Work out the finished part from the listing and answer in its coordinate system (mm). Face numbers are marked on the shaded views. A direction names the side the tool comes from. Coordinates: 2 decimals unless noted, no trailing zeros. Loops run counter-clockwise (first coordinate to the right, second up) from the corner with the lowest first, then second, coordinate; pieces in that order, holes last. Notation, with made-up numbers: (69, 2.25) -> (75, 2.25) arc R14 cw to (75, 14.25) -> close; hole circle Ø9 at (-1.5, 44.5). An arc over 180 degrees is marked (long way). One line per question, with ' | ' between items.
```python
from build123d import *

# Parameters (mm, degrees)
BOSS_EXTRUDE3_DEPTH = 25
BOSS_EXTRUDE4_DEPTH = 14
SKETCH9_R           = 14
CUT_EXTRUDE5_DEPTH  = 97
SKETCH10_W          = 12
SKETCH10_H          = 12
CUT_EXTRUDE6_DEPTH  = 97
SKETCH11_R          = 8
BOSS_EXTRUDE5_DEPTH = 14
FILLET3_R           = 14
SKETCH12_R          = 6
CUT_EXTRUDE8_DEPTH  = 54
FILLET4_R           = 3


with BuildPart() as part:
    # Sketch2 → Boss-Extrude3 (new body, symmetric)
    with BuildSketch(Plane.XY):
        with BuildLine():
            Line((0, 0), (55, 0))
            ThreePointArc((55, 0), (78, 23), (101, 0))
            Line((101, 0), (114, 0))
            ThreePointArc((114, 0), (109.720584442, 17.023645986), (97.899748742, 30))
            Line((97.899748742, 30), (58.100251258, 30))
            ThreePointArc((58.100251258, 30), (49.293476177, 21.724076274), (43.721726998, 11))
            Line((43.721726998, 11), (0, 11))
            Line((0, 11), (0, 0))
        make_face()
    extrude(amount=BOSS_EXTRUDE3_DEPTH, both=True)

    # Sketch7 → Boss-Extrude4 (add, symmetric)
    with BuildSketch(Plane.XY):
        with BuildLine():
            Line((114, 0), (114, 72))
            ThreePointArc((114, 72), (95, 91), (76, 72))
            Line((76, 72), (76, 35.944401511))
            ThreePointArc((76, 35.944401511), (66.65391142, 34.165278777), (58.100251258, 30))
            Line((58.100251258, 30), (97.899748742, 30))
            ThreePointArc((97.899748742, 30), (109.720584442, 17.023645986), (114, 0))
        make_face()
    extrude(amount=BOSS_EXTRUDE4_DEPTH, both=True)

    # Sketch9 → Cut-Extrude5 (cut)
    with BuildSketch(Plane.XY.offset(14)):
        with Locations((95, 72)):
            Circle(SKETCH9_R)
    extrude(amount=-CUT_EXTRUDE5_DEPTH, mode=Mode.SUBTRACT)

    # Sketch10 → Cut-Extrude6 (cut)
    with BuildSketch(Plane(origin=(114, 0, 0), x_dir=(0, 0, -1), z_dir=(1, 0, 0))):
        with Locations((0, 85)):
            Rectangle(SKETCH10_W, SKETCH10_H)
    extrude(amount=-CUT_EXTRUDE6_DEPTH, mode=Mode.SUBTRACT)

    # Sketch11 → Boss-Extrude5 (add)
    with BuildSketch(Plane(origin=(0, 11, 0), x_dir=(1, 0, 0), z_dir=(0, 1, 0))):
        with Locations((19, 0)):
            Circle(SKETCH11_R)
    extrude(amount=BOSS_EXTRUDE5_DEPTH)

    # Fillet3
    fillet3_edges = [part.edges().sort_by_distance(p)[0] for p in [
        (0, 5.5, -25),
        (0, 5.5, 25),
    ]]
    fillet(fillet3_edges, radius=FILLET3_R)

    # Sketch12 → Cut-Extrude8 (cut)
    with BuildSketch(Plane(origin=(0, 25, 0), x_dir=(1, 0, 0), z_dir=(0, 1, 0))):
        with Locations((19, 0)):
            Circle(SKETCH12_R)
    extrude(amount=-CUT_EXTRUDE8_DEPTH, mode=Mode.SUBTRACT)

    # Fillet4
    fillet4_edges = [part.edges().sort_by_distance(p)[0] for p in [
        (43.721726998, 11, 0),
        (11, 11, 0),
    ]]
    fillet(fillet4_edges, radius=FILLET4_R)


solid = part.part
```
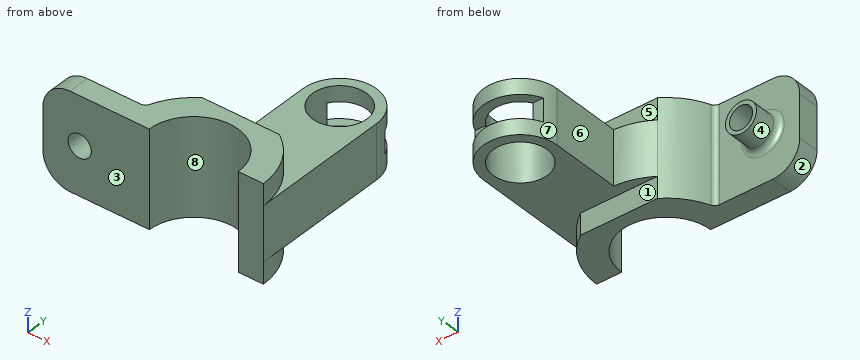
1) For the marked faces 1, 2, 3, 4 and 5, determine the directions among +Z, -Z, +X, -X, +Y, -Y from which every point of the face is accessible in a straight line to the end or side of a thin tool.
Check values:
face 1: -Z, +X, -X, +Y | face 2: -Z, -X, +Y, -Y | face 3: +Z, -Z, +X, -X, -Y | face 4: +Y | face 5: +Z, +X, -X, +Y
2) Find section A-A (y = 65). Write down the section's boundary in (x, z).
Check values:
outline: (76, -14) -> (82.88, -14) -> (82.88, 14) -> (76, 14) -> close; (107.12, -14) -> (114, -14) -> (114, 14) -> (107.12, 14) -> close
3) Find section B-B (z = 0). Write down the section's boundary in (x, y), plus the area to 3 significant figures.
Check values:
outline: (0, 0) -> (13, 0) -> (13, 25) -> (11, 25) -> (11, 14) arc R3 cw to (8, 11) -> (0, 11) -> close; (25, 0) -> (55, 0) arc R23 cw to (101, 0) -> (114, 0) -> (114, 72) arc R19 ccw to (112.66, 79) -> (107.12, 79) arc R14 cw (long way) to (82.88, 79) -> (77.34, 79) arc R19 ccw to (76, 72) -> (76, 35.94) arc R36 ccw to (44.4, 12.92) arc R3 cw to (41.6, 11) -> (30, 11) arc R3 cw to (27, 14) -> (27, 25) -> (25, 25) -> close | area: 3,010 mm^2
4) Flat-ended cylindrical pins translate along their axes: pin 1 (13 mm diameter, centred on x = 17, z = -1, fed in from +Y); pin 2 (12 mm diameter, centred on y = 24.5, z = 1, fed in from -X); pin 3 (4 mm diameter, centred on x = 98, y = 52.5, fed in from -Z); pin 4 (7 mm diameter, centred on x = 19, z = 0, fed in from -Y). Find the tip coordinate at first contact, or state that the pin passes through.
Check values:
pin 1: stops at y = 25 | pin 2: stops at x = 11 | pin 3: stops at z = -14 | pin 4: passes through
5) Find section D-D (x = 104.5). Write down the section's boundary in (y, z).
Check values:
outline: (0, -25) -> (24.37, -25) -> (24.37, -14) -> (61.72, -14) -> (61.72, 14) -> (24.37, 14) -> (24.37, 25) -> (0, 25) -> close; (82.28, -14) -> (88.45, -14) -> (88.45, -6) -> (82.28, -6) -> close; (82.28, 6) -> (88.45, 6) -> (88.45, 14) -> (82.28, 14) -> close
6) Find section C-C (x = 19). Write down the section's boundary in (y, z).
Check values:
outline: (0, -25) -> (11, -25) -> (11, -11) arc R3 cw to (14, -8) -> (25, -8) -> (25, -6) -> (0, -6) -> close; (0, 6) -> (25, 6) -> (25, 8) -> (14, 8) arc R3 cw to (11, 11) -> (11, 25) -> (0, 25) -> close
7) Find the intervals of material crossed by line 1 along X through (y, z) = (14.75, 0); line 2 along X through (y, z) = (21, 1.5); line 3 along Y through (x, z) = (21.5, -13), in increasing order.
Check values:
line 1: x = 11 to 13, 25 to 27, 45.16 to 60.35, 95.65 to 114 | line 2: x = 11.14 to 13.19, 24.81 to 26.86, 48.76 to 68.62, 87.38 to 114 | line 3: y = 0 to 11
8) The mould has two halves that part along X. Classify the marked faces 6, 7 and 8: released by +X, released by -X, zero draft, split by the parting line, or undercut.
Check values:
face 6: released by -X | face 7: split by the parting line | face 8: undercut
